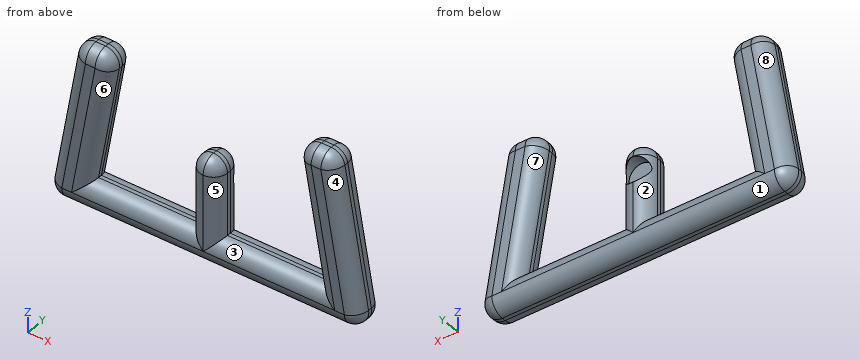
```python
from build123d import *

# Parameters (mm, degrees)
F1_DEPTH = 25
F2_R     = 10.99999
F3_R     = 10
F4_DEPTH = 9.1


# Not quite as in the source:
# - a fillet or chamfer is up to 0.001 mm smaller than in the source, because OpenCascade refuses the exact size


with BuildPart() as f1:
    # F0 (on Front) → F1 (new body)
    with BuildSketch(Plane.XZ):
        Polygon((-104.7428149239, 128.0250078916), (-127.3170780206, 0), (122.4413091306, 0), (99.8670460339, 128.0250078916), (92.5590772594, 128.0250078916), (69.8670460339, 128.0250078916), (88.562115555, 22), (8.562115555, 22), (8.562115555, 82), (-13.437884445, 82), (-13.437884445, 22), (-93.437884445, 22), (-74.7428149239, 128.0250078916), (-93.565618156, 128.0250078916), align=None)
    extrude(amount=F1_DEPTH)

    # F2 (radius 11 in the source; OpenCascade refuses exactly that, so slightly less here)
    f2_edges = [f1.edges().sort_by_distance(p)[0] for p in [
        (-89.742815, -25, 128.025008),
        (-116.029946, -25, 64.012504),
        (-2.437884, -25, 0),
        (111.154178, -25, 64.012504),
        (84.867046, -25, 128.025008),
        (79.214581, -25, 75.012504),
        (48.562116, -25, 22),
        (8.562116, -25, 52),
        (-2.437884, -25, 82),
        (-13.437884, -25, 52),
        (-53.437884, -25, 22),
        (-84.09035, -25, 75.012504),
        (-89.742815, 0, 128.025008),
        (-116.029946, 0, 64.012504),
        (-2.437884, 0, 0),
        (111.154178, 0, 64.012504),
        (84.867046, 0, 128.025008),
        (79.214581, 0, 75.012504),
        (48.562116, 0, 22),
        (8.562116, 0, 52),
        (-2.437884, 0, 82),
        (-13.437884, 0, 52),
        (-53.437884, 0, 22),
        (-84.09035, 0, 75.012504),
        (-74.742815, -12.5, 128.025008),
        (-104.742815, -12.5, 128.025008),
        (8.562116, -12.5, 82),
        (-13.437884, -12.5, 82),
        (99.867046, -12.5, 128.025008),
        (69.867046, -12.5, 128.025008),
        (122.441309, -12.5, 0),
        (-127.317078, -12.5, 0),
    ]]
    fillet(f2_edges, radius=F2_R)

    # F3 (on Front) → F4 (cut)
    with BuildSketch(Plane.XZ):
        with Locations((-2.4443906732, 60.8239136636)):
            Circle(F3_R)
    extrude(amount=F4_DEPTH, mode=Mode.SUBTRACT)


solid = f1.part
```
Verification items for the finished model (mm, model axes). Face numbers are marked on the shaded views. A direction names the side the tool comes from. Round coordinates to 2 decimals unless told otherwise and drop trailing zeros. Write each question's results on one line, items separated by ' | '. Start each with the question number.
1. Draft check along X on the marked faces 1, 2, 3 and 4. Enter one of: +X half, -X half, draft (parallel to the pull), parting line (faces both ways), or undercut.
2. Material ranges on probe 1 along X at (y, z) = (-21.75, 77); probe 2 along X at (y, z) = (-8.5, 58); probe 3 along X at (y, z) = (-15.75, 75.5), recorded low to high. Write a range as from..to.
3. Depth check by flat-ended pin: P1, Ø0.9, axis at y = -13, z = 52.5, coming from the -X side; P2, Ø2, axis at x = -42, z = 15, coming from the +Y side; P3, Ø6, axis at y = -10, z = 108, coming from the -X side. Enter the tip coordinate at first touch or a pass-through.
4. Set-up check for the marked faces 5, 6, 7 and 8: record each of +Z, -Z, +X, -X, +Y, -Y from which the full face is reachable in a straight line by a thin tool's end or side.
Solutions:
1) face 1: draft | face 2: undercut | face 3: undercut | face 4: +X half
2) probe 1: x = -110.5..-86.98, -7.43..2.56, 82.11..105.62 | probe 2: x = -116.8..-87.38, -13.15..-12.04, 7.15..8.27, 82.51..111.92 | probe 3: x = -113.86..-84.15, -12.32..7.45, 79.27..108.99
3) P1: stops at x = -118.14 | P2: stops at y = -0.42 | P3: stops at x = -108.78
4) face 5: +Z, -Y | face 6: -Y | face 7: +Y | face 8: +Z, -X, +Y
